from build123d import *

# Parameters (mm, degrees)
F0_W        = 100
F0_H        = 100
F1_DEPTH    = 2
F2_W        = 15
F2_H        = 15
F3_DEPTH    = 15
F4_T        = 2
F4_T3_DEPTH = 19
F4_T5_DEPTH = 19
F4_T7_DEPTH = 19
F4_T9_DEPTH = 19
F6_DEPTH    = 2.001


# Not quite as in the source:
# - a shell that OpenCascade refuses in one call is made with other operations: the cavity is built on its own and cut out


with BuildPart() as f1:
    # F0 (on Top) → F1 (new body)
    with BuildSketch(Plane.XY):
        Rectangle(F0_W, F0_H)
    extrude(amount=F1_DEPTH)

    # F2 (on face) → F3 (join)
    with BuildSketch(Plane.XY.offset(2)):
        with Locations((-42.5, -42.5)):
            Rectangle(F2_W, F2_H)
        with Locations((-42.5, 42.5)):
            Rectangle(F2_W, F2_H)
        with Locations((42.5, 42.5)):
            Rectangle(F2_W, F2_H)
        with Locations((42.5, -42.5)):
            Rectangle(F2_W, F2_H)
    extrude(amount=F3_DEPTH)

    # F4: shell of thickness 2, made by hand


with BuildPart() as f4_core1:
    # F4_t2: copy of F1
    add(f1.part)

    # the walls: a layer under each face that stays
    f4_faces = [f4_core1.faces().sort_by_distance(p)[0] for p in [
        (50, -42.8571428571, 15.7857142857),
        (0, 0, 0),
        (-50, 42.8571428571, 15.7857142857),
        (-35, -42.5, 9.5),
        (-42.5, -35, 9.5),
        (-42.5, 35, 9.5),
        (-35, 42.5, 9.5),
        (42.8571428571, 50, 15.7857142857),
        (35, 42.5, 9.5),
        (42.5, 35, 9.5),
        (0, 0, 2),
        (35, -42.5, 9.5),
        (42.5, -35, 9.5),
        (-42.8571428571, -50, 15.7857142857),
    ]]
    thicken(f4_faces, amount=-F4_T, mode=Mode.SUBTRACT)

    # F4_s4 → F4_t3 (cut)
    with BuildSketch(Plane.XZ.offset(33)):
        Polygon((-34.98, 2.02), (-37, 2), (-37, 0), (-35, 0), align=None)
        Polygon((34.98, 2.02), (35, 0), (37, 0), (37, 2), align=None)
    extrude(amount=F4_T3_DEPTH, mode=Mode.SUBTRACT)

    # F4_s6 → F4_t5 (cut)
    with BuildSketch(Plane.YZ.offset(-52)):
        Polygon((-34.98, 2.02), (-37, 2), (-37, 0), (-35, 0), align=None)
        Polygon((34.98, 2.02), (37, 2), (37, 0), (35, 0), align=None)
    extrude(amount=F4_T5_DEPTH, mode=Mode.SUBTRACT)

    # F4_s8 → F4_t7 (cut)
    with BuildSketch(Plane.XZ.offset(-52)):
        Polygon((-34.98, 2.02), (-37, 2), (-37, 0), (-35, 0), align=None)
        Polygon((34.98, 2.02), (37, 2), (37, 0), (35, 0), align=None)
    extrude(amount=F4_T7_DEPTH, mode=Mode.SUBTRACT)

    # F4_s10 → F4_t9 (cut)
    with BuildSketch(Plane.YZ.offset(33)):
        Polygon((34.98, 2.02), (37, 2), (37, 0), (35, 0), align=None)
        Polygon((-34.98, 2.02), (-35, 0), (-37, 0), (-37, 2), align=None)
    extrude(amount=F4_T9_DEPTH, mode=Mode.SUBTRACT)


with BuildPart() as f1_1:
    add(f1.part)

    # what is left inside the walls is the cavity
    f4_cavity = [f4_core1.part.solids().sort_by_distance(p)[0] for p in [
        (47.98, -42.5, 12),
        (47.98, 42.5, 12),
        (-42.5, -47.98, 12),
        (-37.02, 42.5, 12),
    ]]
    add(f4_cavity, mode=Mode.SUBTRACT)

    # F5 (on face) → F6 (cut, through all)
    with BuildSketch(Plane.XY.offset(2)):
        with BuildLine():
            Line((-30.0000010431, -45.0000010431), (30.0000010431, -45.0000010431))
            Line((30.0000010431, -45.0000010431), (30.0000010431, -33.535534949))
            Line((30.0000010431, -33.535534949), (1.2940952255, -4.8296291314))
            ThreePointArc((1.2940952255, -4.8296291314), (0, -5), (-1.2940952255, -4.8296291314))
            Line((-1.2940952255, -4.8296291314), (-30.0000010431, -33.535534949))
            Line((-30.0000010431, -33.535534949), (-30.0000010431, -45.0000010431))
        make_face()
        with BuildLine():
            Line((-33.535534949, 30.0000010431), (-45.0000010431, 30.0000010431))
            Line((-45.0000010431, 30.0000010431), (-45.0000010431, -30.0000010431))
            Line((-45.0000010431, -30.0000010431), (-33.535534949, -30.0000010431))
            Line((-33.535534949, -30.0000010431), (-4.8296291314, -1.2940952255))
            ThreePointArc((-4.8296291314, -1.2940952255), (-5, 0), (-4.8296291314, 1.2940952255))
            Line((-4.8296291314, 1.2940952255), (-33.535534949, 30.0000010431))
        make_face()
        with BuildLine():
            Line((30.0000010431, 45.0000010431), (-30.0000010431, 45.0000010431))
            Line((-30.0000010431, 45.0000010431), (-30.0000010431, 33.535534949))
            Line((-30.0000010431, 33.535534949), (-1.2940952255, 4.8296291314))
            ThreePointArc((-1.2940952255, 4.8296291314), (0, 5), (1.2940952255, 4.8296291314))
            Line((1.2940952255, 4.8296291314), (30.0000010431, 33.535534949))
            Line((30.0000010431, 33.535534949), (30.0000010431, 45.0000010431))
        make_face()
        with BuildLine():
            Line((45.0000010431, -30.0000010431), (45.0000010431, 30.0000010431))
            Line((45.0000010431, 30.0000010431), (33.535534949, 30.0000010431))
            Line((33.535534949, 30.0000010431), (4.8296291314, 1.2940952255))
            ThreePointArc((4.8296291314, 1.2940952255), (5, 0), (4.8296291314, -1.2940952255))
            Line((4.8296291314, -1.2940952255), (33.535534949, -30.0000010431))
            Line((33.535534949, -30.0000010431), (45.0000010431, -30.0000010431))
        make_face()
    extrude(amount=-F6_DEPTH, mode=Mode.SUBTRACT)


solid = f1_1.part
Work out the finished part from the listing and answer in its coordinate system (mm). A direction names the side the tool comes from. Coordinates: 2 decimals unless noted, no trailing zeros. Loops run counter-clockwise (first coordinate to the right, second up) from the corner with the lowest first, then second, coordinate; pieces in that order, holes last. Notation, with made-up numbers: (3, 58.5) -> (46, 58.5) arc R25 cw to (46, 90.5) -> close; hole circle Ø6 at (48, 79.25). An arc over 180 degrees is marked (long way). Write each question's results on one line, items separated by ' | '. Start each with the question number.
1) Flat-ended cylindrical pins translate along their axes: P1, Ø3.5, axis at x = 43.5, y = -41.5, coming from the +Z side; P2, Ø12, axis at x = -45, y = -41, coming from the +Z side. Find the tip coordinate at first contact, or state that the pin passes through.
2) Find section A-A on z = 6. Count the separate pieces of the cut face and the enclosed holes in it, then the cut area to 3 significant figures.
3) For faces 4 (the flat face through (-43, -35, 9)), 5 (the flat face through (-15.848, 19.384, 1.014)), 6 (the flat face through (-37, 42, 9)), determine the directions among +Z, -Z, +X, -X, +Y, -Y from which every point of the face is accessible in a straight line to the end or side of a thin tool.
4) Find section B-B on y = 41.5. Determine the outline of the cut face in (x, z), then the cut area to 3 significant figures.
5) Consider line 1 along Y through (x, z) = (-40, 16.25); line 2 along Y through (x, z) = (-36, 5); line 3 along Y through (x, z) = (-25.5, 1.5). Determine where each line is inside the solid, lowest interval first.
6) The mould has two halves that part along X. Classify faces 1 (the flat face through (-43, 48, 9)), 2 (the flat face through (50, -0.2, 0.3)), 3 (the flat face through (-50, -0.2, 0.3)): pulls with the +X half, pulls with the -X half, needs draft (parallel to the pull), parting line crosses it, or undercut.
7) Find section D-D on x = 13.5. Determine the outline of the cut face in (y, z).
Response values:
1) P1: stops at z = 2 | P2: stops at z = 17
2) separate pieces: 4 | enclosed holes: 4 | area: 416 mm^2
3) face 4: +Z, +X, -X | face 5: +Z, -Z | face 6: +Z
4) outline: (-50, 0) -> (-30, 0) -> (-30, 2) -> (-35, 2) -> (-35, 17) -> (-37, 17) -> (-37, 2) -> (-48, 2) -> (-48, 17) -> (-50, 17) -> close; (30, 0) -> (50, 0) -> (50, 17) -> (48, 17) -> (48, 2) -> (37, 2) -> (37, 17) -> (35, 17) -> (35, 2) -> (30, 2) -> close | area: 200 mm^2
5) line 1: y = -50 to -48, -37 to -35, 35 to 37, 48 to 50 | line 2: y = -50 to -35, 35 to 50 | line 3: y = -50 to -45, -29.04 to -21.96, 21.96 to 29.04, 45 to 50
6) face 1: undercut | face 2: pulls with the +X half | face 3: pulls with the -X half
7) outline: (-50, 0) -> (-45, 0) -> (-45, 2) -> (-50, 2) -> close; (-17.04, 0) -> (-9.96, 0) -> (-9.96, 2) -> (-17.04, 2) -> close; (9.96, 0) -> (17.04, 0) -> (17.04, 2) -> (9.96, 2) -> close; (45, 0) -> (50, 0) -> (50, 2) -> (45, 2) -> close
